Work out the finished part from the listing and answer in its coordinate system (mm). Face numbers are marked on the shaded views. A direction names the side the tool comes from. Coordinates: 2 decimals unless noted, no trailing zeros. Order: outer loops, then holes, each group sorted by start corner. A loop starts at its lowest first (then second) coordinate and runs counter-clockwise, first axis right, second up. Notation, with made-up numbers: M 75,18.25 L 103,18.25 A23 ccw 103,37.25 Z; hole C 7,-14 d6. An arc over 180 degrees is marked long. Write item = value, one per line. Start each with the question number.
Q1. Determine the mould class of the marked faces 1, 2, 3 and 4 for opening direction X: released by +X, released by -X, zero draft, split by the parting line, or undercut.
Q2. A tool of negligible diameter and unlimited length cuts with its end or side. For the marked faces 5, 6, 7, 8 and 9, from which of +Z, -Z, +X, -X, +Y, -Y can it reach the whole face along a straight path? Write none if from no direction.
Q3. Find section B-B on z = 2.5. Give the vertices of the cut face in (x, y).
Q4. Each of these flat-tipped pins is pushed along its axis until it touches: P1, Ø6.5, axis at y = 18, z = 8, coming from the +X side; P2, Ø2, axis at x = -4.5, y = 11.5, coming from the -Z side; P3, Ø3, axis at x = -19.5, z = 8.5, coming from the +Y side; P4, Ø5, axis at y = -15.5, z = 11, coming from the -X side. Where does it stop, or does it pass through?
Q5. Straight lines are drawn through the part: line 1 along X through (y, z) = (15.5, 3); line 2 along Y through (x, z) = (-11.5, 5.5); line 3 along X through (y, z) = (8.5, 6). For each, find the intervals that lie inside material, in ascending order.
Q6. Find section C-C on y = 10.5. Give the vertices of the cut face in (x, z).
Q7. Find section D-D on x = -16.5. Give the vertices of the cut face in (y, z).
Q8. Find section A-A on z = 6.35. Give the vertices of the cut face in (x, y).
```python
from build123d import *

# Parameters (mm, degrees)
F1_DEPTH = 12.7
F2_W     = 2.54
F2_H     = 12.7
F3_DEPTH = 12.7
F4_R     = 1.27
F5_DEPTH = 25.4
F6_R     = 1.27
F7_DEPTH = 25.4
F8_R     = 5.08


with BuildPart() as f1:
    # F0 (on Top) → F1 (new body)
    with BuildSketch(Plane.XY):
        Polygon((-25.4, 14.664697), (0, -29.329394), (25.4, 14.664697), align=None)
    extrude(amount=F1_DEPTH)

    # F2 (on face) → F3 (join)
    with BuildSketch(Plane(origin=(0, 14.664697, 0), x_dir=(-1, 0, 0), z_dir=(0, 1, 0))):
        with Locations((-13.97, 6.35)):
            Rectangle(F2_W, F2_H)
        with Locations((13.97, 6.35)):
            Rectangle(F2_W, F2_H)
    extrude(amount=F3_DEPTH)

    # F4 (on face) → F5 (cut)
    with BuildSketch(Plane.YZ.offset(15.24)):
        with Locations((21.014697, 6.35)):
            Circle(F4_R)
    extrude(amount=-F5_DEPTH, mode=Mode.SUBTRACT)

    # F6 (on face) → F7 (cut)
    with BuildSketch(Plane(origin=(-15.24, 0, 0), x_dir=(0, -1, 0), z_dir=(-1, 0, 0))):
        with Locations((-21.014697, 6.35)):
            Circle(F6_R)
    extrude(amount=-F7_DEPTH, mode=Mode.SUBTRACT)

    # F8
    f8_edges = [f1.edges().sort_by_distance(p)[0] for p in [
        (13.97, 27.364697, 12.7),
        (13.97, 27.364697, 0),
        (-13.97, 27.364697, 12.7),
        (-13.97, 27.364697, 0),
    ]]
    fillet(f8_edges, radius=F8_R)


solid = f1.part
```
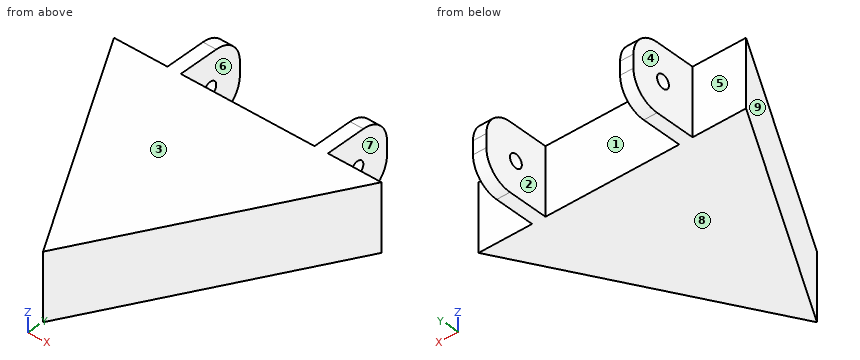
Findings below:
q1.face_1 = undercut
q1.face_2 = undercut
q1.face_3 = zero draft
q1.face_4 = released by -X
q2.face_5 = +Z, -Z, -X, +Y
q2.face_6 = +Z, -Z, +Y
q2.face_7 = +Z, -Z, +X, +Y
q2.face_8 = -Z, +X, -X, +Y, -Y
q2.face_9 = +Z, -Z, -X, -Y
q3.outline = M -25.4,14.66 L 0,-29.33 L 25.4,14.66 L 15.24,14.66 L 15.24,26.66 L 12.7,26.66 L 12.7,14.66 L -12.7,14.66 L -12.7,26.66 L -15.24,26.66 L -15.24,14.66 Z
q4.P1 = 15.24
q4.P2 = 0
q4.P3 = 14.66
q4.P4 = -9.43
q5.line_1 = -15.24 to -12.7, 12.7 to 15.24
q5.line_2 = -9.41 to 14.66
q5.line_3 = -21.84 to 21.84
q6.outline = M -23,0 L 23,0 L 23,12.7 L -23,12.7 Z
q7.outline = M -0.75,0 L 14.66,0 L 14.66,12.7 L -0.75,12.7 Z
q8.outline = M -25.4,14.66 L 0,-29.33 L 25.4,14.66 L 15.24,14.66 L 15.24,19.74 L 12.7,19.74 L 12.7,14.66 L -12.7,14.66 L -12.7,19.74 L -15.24,19.74 L -15.24,14.66 Z; M -15.24,22.28 L -12.7,22.28 L -12.7,27.36 L -15.24,27.36 Z; M 12.7,22.28 L 15.24,22.28 L 15.24,27.36 L 12.7,27.36 Z
